Autodesk Fusion 360 part; units mm, degrees
sketch "스케치1" plane through (0, 0, 0) normal (0, 0, 1) x (1, 0, 0)
sketch "스케치2" plane through (0, 0, 0) normal (0, 0, 1) x (1, 0, 0)
  circle A0 centre (0, 0) radius 35
  dimension "d1" = 70
extrude "돌출1" add sketch "스케치2" along normal blind 100 draft 7
shell "쉘1" thickness 3 removed faces 1 at (-3.1952, -13.2971, 100)
fillet "필렛1" radius 1.4 2 edges at (-44.079, 17.0966, 100) (-41.261, 16.0036, 100)
fillet "필렛2" radius 4 2 edges at (-32.6315, -12.6565, 0) (-30.1569, -11.6967, 3)
CAD build for the part. Positions are in the model's coordinates, mm. Coordinates: 2 decimals unless noted, no trailing zeros. Write each loop counter-clockwise with the first axis right and the second up, starting at its lowest first coordinate (ties: lowest second). Pieces come first, ordered by that corner, then holes. Notation, with made-up numbers: (-23.75, 77) -> (0.25, 77) arc R20 cw to (0.25, 93) -> close; hole circle Ø2 at (-27.75, 9). An arc over 180 degrees is marked (long way). Use CSV: the item, a comma, the result in double quotes. Start each with the question number.
Item 1: Band-saw the part on A-A, the plane x = 0. Write the cut outline in (y, z), plus the area to 3 significant figures.
Item 2: Wall check: probe 1 along X at (y, z) = (-6.5, 6); probe 2 along X at (y, z) = (-33.5, 78); probe 3 along Y at (x, z) = (13.5, 61). Give the ranges that are in metal, low to high.
Item 3: Two-plate mould, pull along X, no slides. Class faces 1 (the flat face through (0, 0, 0)), 2 (the conical face through (-30.6, -23.4, 53.3)), 3 (the conical face through (39.43, 12.42, 51.64)): +X half, -X half, draft (parallel to the pull), parting line (faces both ways), or undercut.
Item 4: Band-saw the part on D-D, the plane z = 50.5. Write the cut outline in (x, y).
Item 5: Band-saw the part on C-C, the plane z = 22.5. Write the cut outline in (x, y).
Item 6: Drop flat-ended pins along their axis: P1, Ø2, axis at y = 27, z = 66.5, coming from the +X side; P2, Ø10, axis at x = -14, z = 67, coming from the +Y side; P3, Ø8, axis at y = -26, z = 52, coming from the -X side. Give the stop position or say it passes through.
Response values:
1,outline,"(-47.09, 98.43) -> (-35.43, 3.51) arc R4 ccw to (-31.46, 0) -> (31.46, 0) arc R4 ccw to (35.43, 3.51) -> (47.09, 98.43) arc R1.4 ccw to (45.7, 100) -> (45.49, 100) arc R1.4 ccw to (44.1, 98.77) -> (32.78, 6.51) arc R4 cw to (28.81, 3) -> (-28.81, 3) arc R4 cw to (-32.78, 6.51) -> (-44.1, 98.77) arc R1.4 ccw to (-45.49, 100) -> (-45.7, 100) arc R1.4 ccw to start"
1,area,"796 mm2"
2,probe 1,"x = -35.14 to -32.03, 32.03 to 35.14"
2,probe 2,"x = -29.41 to -24.59, 24.59 to 29.41"
2,probe 3,"y = -40.29 to -37.09, 37.09 to 40.29"
3,face 1,"draft"
3,face 2,"undercut"
3,face 3,"parting line"
4,outline,"circle Ø82.4 at (0, 0); hole circle Ø76.36 at (0, 0)"
5,outline,"circle Ø75.53 at (0, 0); hole circle Ø69.48 at (0, 0)"
6,P1,"stops at x = 34.47"
6,P2,"stops at y = 42.45"
6,P3,"stops at x = -35.12"
